```python
from build123d import *

# Parameters (mm, degrees)
CROQUIS1_W              = 17
CROQUIS1_H              = 27
SALIENTE_EXTRUIR1_DEPTH = 0.5
CROQUIS2_R              = 1.2
CORTAR_EXTRUIR1_DEPTH   = 0.5
CROQUIS3_W              = 1.387036679
CROQUIS3_H              = 1.014497707
CROQUIS3_H_2            = 0.94749306
CROQUIS3_W_2            = 1.216641307
CROQUIS3_H_3            = 3.776719189
CROQUIS3_W_3            = 3.892395648
CROQUIS3_H_4            = 1.091909055
SALIENTE_EXTRUIR2_DEPTH = 0.5


with BuildPart() as part:
    # Croquis1 → Saliente-Extruir1 (new body)
    with BuildSketch(Plane.XY):
        with Locations((8.5, 13.5)):
            Rectangle(CROQUIS1_W, CROQUIS1_H)
    extrude(amount=SALIENTE_EXTRUIR1_DEPTH)

    # Croquis2 → Cortar-Extruir1 (cut)
    with BuildSketch(Plane.XY.offset(0.5)):
        with Locations((2, 2)):
            Circle(CROQUIS2_R)
        with Locations((15, 25)):
            Circle(CROQUIS2_R)
    extrude(amount=-CORTAR_EXTRUIR1_DEPTH, mode=Mode.SUBTRACT)

    # Croquis3 → Saliente-Extruir2 (add)
    with BuildSketch(Plane.XY.offset(0.5)):
        with Locations((3.960596796, 20.650173654)):
            Rectangle(CROQUIS3_W, CROQUIS3_H)
        with Locations((3.960596796, 17.670424265)):
            Rectangle(CROQUIS3_W, CROQUIS3_H_2)
        with Locations((10.721614084, 13.296281172)):
            Rectangle(CROQUIS3_W_2, CROQUIS3_H_3)
        with Locations((5.588615761, 6.764486289)):
            Rectangle(CROQUIS3_W_3, CROQUIS3_H_4)
    extrude(amount=SALIENTE_EXTRUIR2_DEPTH)


solid = part.part
```
Could you check a few things on this model? Use its own coordinates, in mm. Round coordinates to 2 decimals unless told otherwise and drop trailing zeros. Loops run counter-clockwise (first coordinate to the right, second up) from the corner with the lowest first, then second, coordinate; pieces in that order, holes last. Notation, with made-up numbers: (50, -17) - (104, -17) arc R22 ccw to (104, 13) - close; hole circle Ø11 at (-5.75, 9.5). An arc over 180 degrees is marked (long way). Answer in a Markdown table with one row per item. Add a question column.
(1) I'm going to push flat-ended pins straight in: pin 1 (0.6 mm diameter, centred on x = 4, z = 1, fed in from +Y); pin 2 (1.5 mm diameter, centred on x = 5.5, y = 22, fed in from -Z). Where does each tip first touch, or does it pass through?
(2) If we mould it in two halves opening along Y, with no side actions, what happens to faces 1 (the face through (4, 21, 1)), 2 (the face through (2.65, 3.01, 0.25)), 3 (the face through (15.554, 23.935, 0.254))? For each: pulls with the +Y half, pulls with the -Y half, needs draft (parallel to the pull), parting line crosses it, or undercut.
(3) If we section it at D-D (y = 13.25): Please give me the cut outline in (x, z).
(4) If we section it at C-C (y = 2): Please give me the cut outline in (x, z), plus the area to 3 significant figures.
(5) If we section it at A-A (x = 2): Please give me the cut outline in (y, z).
(6) If we section it at B-B (z = 0.65): Please give me the cut outline in (x, y).
(7) I need wall thicknesses on line 1 along Y through (x, z) = (2, 0.25); line 2 along Y through (x, z) = (15, 0.1); line 3 along Z through (x, y) = (6.75, 25). Which ranges of each line are inside material? Lowest first, please.
Model answer:
| question | item | result |
|---|---|---|
| 1 | pin 1 | stops at y = 21.16 |
| 1 | pin 2 | stops at z = 0 |
| 2 | face 1 | needs draft |
| 2 | face 2 | undercut |
| 2 | face 3 | undercut |
| 3 | outline | (0, 0) - (17, 0) - (17, 0.5) - (11.33, 0.5) - (11.33, 1) - (10.11, 1) - (10.11, 0.5) - (0, 0.5) - close |
| 4 | outline | (0, 0) - (0.8, 0) - (0.8, 0.5) - (0, 0.5) - close; (3.2, 0) - (17, 0) - (17, 0.5) - (3.2, 0.5) - close |
| 4 | area | 7.30 mm² |
| 5 | outline | (0, 0) - (0.8, 0) - (0.8, 0.5) - (0, 0.5) - close; (3.2, 0) - (27, 0) - (27, 0.5) - (3.2, 0.5) - close |
| 6 | outline | (3.27, 17.2) - (4.65, 17.2) - (4.65, 18.14) - (3.27, 18.14) - close; (3.27, 20.14) - (4.65, 20.14) - (4.65, 21.16) - (3.27, 21.16) - close; (3.64, 6.22) - (7.53, 6.22) - (7.53, 7.31) - (3.64, 7.31) - close; (10.11, 11.41) - (11.33, 11.41) - (11.33, 15.18) - (10.11, 15.18) - close |
| 7 | line 1 | y = 0 to 0.8, 3.2 to 27 |
| 7 | line 2 | y = 0 to 23.8, 26.2 to 27 |
| 7 | line 3 | z = 0 to 0.5 |
